from build123d import *

# Parameters (mm, degrees)
BOSS_EXTRUDE2_DEPTH = 20
SKETCH4_R           = 1.05
CUT_EXTRUDE1_DEPTH  = 5.479855617


with BuildPart() as part:
    # Sketch2 → Boss-Extrude2 (new body)
    with BuildSketch(Plane.XY):
        Polygon((0, 0), (2.5, 0), (4.600215416, 9), (2.100215416, 9), align=None)
    extrude(amount=BOSS_EXTRUDE2_DEPTH)

    # Sketch4 → Cut-Extrude1 (cut, through all)
    with BuildSketch(Plane(origin=(0, 0, 0), x_dir=(0, 0, 1), z_dir=(-0.973836052, 0.227251721, 0))):
        with Locations((3.625, 3.2)):
            Circle(SKETCH4_R)
        with Locations((16.375, 3.2)):
            Circle(SKETCH4_R)
    extrude(amount=-CUT_EXTRUDE1_DEPTH, mode=Mode.SUBTRACT)


solid = part.part
Source: CAD feature listing. Evaluate the final solid. Frame: model axes, mm. Give positions to 0.01 mm unless a question says otherwise; leave off trailing zeros. Write each loop counter-clockwise with the first axis right and the second up, starting at its lowest first coordinate (ties: lowest second). Pieces come first, ordered by that corner, then holes. Notation, with made-up numbers: (4, 79) -> (26, 79) arc R32 cw to (26, 111) -> close; hole circle Ø6 at (41.25, -13.5). An arc over 180 degrees is marked (long way). Return JSON: item names as keys, results as strings. Group by question number.
1. Pin query (flat end, axial travel): pin 1 Ø3 at (y, z) = (5.5, 9.5) entering from +X; pin 2 Ø4 at (y, z) = (2.5, 2) entering from -X; pin 3 Ø5 at (y, z) = (5.5, 8) entering from +X. Return the tip coordinate at first contact, or that it passes through.
2. Section A-A, the plane z = 6.25. Output: boundary loops of the cut face in (x, y).
3. Mould query, pull axis Y, two halves, no side actions, for faces 1 (the face through (1.065, 4.563, 9.86)), 2 (the face through (2, 5, 20)), 3 (the face through (1.907, 2.888, 2.576)), 4 (the face through (1, 0, 10)). Classes: +Y half, -Y half, draft (parallel to the pull), parting line (faces both ways), or undercut.
4. Material intervals for line 1 (Z direction, x = 2, y = 2); line 2 (Z direction, x = 1.05, y = 4); line 3 (X direction, y = 6.25, z = 14.5), sorted ascending. Write a range as from..to.
5. Section B-B, the plane x = 4.05. Output: boundary loops of the cut face in (y, z).
6. Section C-C, the plane x = 1.65. Count the separate pieces of the cut face and the enclosed holes in it, then the cut area to 3 significant figures.
Determined:
{
 "1": {"pin 1": "stops at x = 4.13", "pin 2": "stops at x = 0.12", "pin 3": "stops at x = 4.37"},
 "2": {"outline": "(0, 0) -> (2.5, 0) -> (4.6, 9) -> (2.1, 9) -> close"},
 "3": {"face 1": "+Y half", "face 2": "draft", "face 3": "undercut", "face 4": "-Y half"},
 "4": {"line 1": "z = 0..2.94, 4.31..15.69, 17.06..20", "line 2": "z = 0..3.15, 4.1..15.9, 16.85..20", "line 3": "x = 1.46..3.96"},
 "5": {"outline": "(6.64, 0) -> (9, 0) -> (9, 20) -> (6.64, 20) -> close"},
 "6": {"separate pieces": "1", "enclosed holes": "2", "area": "134 mm2"}
}
